```python
from build123d import *

# Parameters (mm, degrees)
AUFSATZ_LINEAR_AUSTRAGEN1_DEPTH      = 10
AUFSATZ_LINEAR_AUSTRAGEN1_DEPTH_BACK = 10
SKIZZE2_R                            = 2.5
AUFSATZ_LINEAR_AUSTRAGEN2_DEPTH      = 2.5
M3_GEWINDEBOHRUNG1_D                 = 2.5


with BuildPart() as part:
    # Skizze1 → Aufsatz-Linear austragen1 (new, two sides: drawn at the far end of the back side and taken through both)
    with BuildSketch(Plane.XY.offset(-AUFSATZ_LINEAR_AUSTRAGEN1_DEPTH_BACK)):
        Polygon((-7, 0), (7, 0), (7, 1.5), (4.8, 1.5), (4.8, 4), (-4.8, 4), (-4.8, 1.5), (-7, 1.5), align=None)
    extrude(amount=AUFSATZ_LINEAR_AUSTRAGEN1_DEPTH + AUFSATZ_LINEAR_AUSTRAGEN1_DEPTH_BACK)

    # Skizze2 → Aufsatz-Linear austragen2 (add)
    with BuildSketch(Plane(origin=(0, 4, 0), x_dir=(1, 0, 0), z_dir=(0, 1, 0))):
        with Locations(Location((0, 7, 0), (0, 0, 270))):
            Circle(SKIZZE2_R)
        with Locations(Location((0, -7, 0), (0, 0, 270))):
            Circle(SKIZZE2_R)
    extrude(amount=AUFSATZ_LINEAR_AUSTRAGEN2_DEPTH)

    # M3 Gewindebohrung1 (through all)
    with Locations(Plane(origin=(0, 6.5, 0), x_dir=(1, 0, 0), z_dir=(0, 1, 0))):
        with Locations((0, -7), (0, 7)):
            Hole(M3_GEWINDEBOHRUNG1_D / 2)


solid = part.part
```
CAD build for the part. Positions are in the model's coordinates, mm. A direction names the side the tool comes from. Round coordinates to 2 decimals unless told otherwise and drop trailing zeros. Loops run counter-clockwise (first coordinate to the right, second up) from the corner with the lowest first, then second, coordinate; pieces in that order, holes last. Notation, with made-up numbers: M -38,25 L -32,25 A29 cw -32,58 Z; hole C 88.5,82 d1. An arc over 180 degrees is marked long. Return JSON: item names as keys, results as strings. Group by question number.
(1) Mould opens along Z. For faces 4 (the flat face through (0, 2, 10)), 5 (the cylindrical face through (0.751, 5.232, 9.385)), 6 (the flat face through (4.8, 3, 0)) say: +Z half, -Z half, draft (parallel to the pull), parting line (faces both ways), or undercut.
(2) Drop flat-ended pins along their axis: P1, Ø2.5, axis at x = 6.5, z = -3, coming from the +Y side; P2, Ø2, axis at x = 0, z = -7, coming from the -Y side; P3, Ø1.2, axis at y = 3, z = 1, coming from the -X side; P4, Ø4, axis at x = -2.5, z = -3, coming from the +Y side. Give the stop position or say it passes through.
(3) Wall check: probe 1 along Z at (x, y) = (0, 3); probe 2 along X at (y, z) = (4.25, 7); probe 3 along X at (y, z) = (2.25, 7). Give the ranges that are in metal, low to high. Write a range as [from, to].
(4) Saw through at C-C, the plane z = -2. List the corners of the cut face in (x, y), and give its area (3 significant figures).
(5) Tool access for faces 1 (the flat face through (6, 1.5, 0)), 2 (the flat face through (-4.8, 3, 0)), 3 (the flat face through (0, 4, 0)): list every direction of +Z, -Z, +X, -X, +Y, -Y with a clear straight run to the whole face (end or side of a thin tool).
(6) Saw through at B-B, the plane x = 0. List the corners of the cut face in (y, z), and give its area (3 significant figures).
(7) Saw through at A-A, the plane z = 7. List the corners of the cut face in (x, y), and give its area (4 significant figures).
(8) Saw through at D-D, the plane y = 4.5. List the corners of the cut face in (x, z).
Answer list:
{
 "1": {"face 4": "+Z half", "face 5": "undercut", "face 6": "draft"},
 "2": {"P1": "y = 1.5", "P2": "through", "P3": "x = -4.8", "P4": "y = 4"},
 "3": {"probe 1": "[-10, -8.25], [-5.75, 5.75], [8.25, 10]", "probe 2": "[-2.5, -1.25], [1.25, 2.5]", "probe 3": "[-4.8, -1.25], [1.25, 4.8]"},
 "4": {"outline": "M -7,0 L 7,0 L 7,1.5 L 4.8,1.5 L 4.8,4 L -4.8,4 L -4.8,1.5 L -7,1.5 Z", "area": "45.0 mm2"},
 "5": {"face 1": "+Z, -Z, +X, +Y", "face 2": "+Z, -Z, -X, +Y", "face 3": "+Y"},
 "6": {"outline": "M 0,-10 L 4,-10 L 4,-9.5 L 6.5,-9.5 L 6.5,-8.25 L 0,-8.25 Z; M 0,-5.75 L 6.5,-5.75 L 6.5,-4.5 L 4,-4.5 L 4,4.5 L 6.5,4.5 L 6.5,5.75 L 0,5.75 Z; M 0,8.25 L 6.5,8.25 L 6.5,9.5 L 4,9.5 L 4,10 L 0,10 Z", "area": "72.5 mm2"},
 "7": {"outline": "M -7,0 L -1.25,0 L -1.25,6.5 L -2.5,6.5 L -2.5,4 L -4.8,4 L -4.8,1.5 L -7,1.5 Z; M 1.25,0 L 7,0 L 7,1.5 L 4.8,1.5 L 4.8,4 L 2.5,4 L 2.5,6.5 L 1.25,6.5 Z", "area": "41.25 mm2"},
 "8": {"outline": "C 0,-7 d5; C 0,7 d5; hole C 0,-7 d2.5; hole C 0,7 d2.5"}
}
